Design review of the part built by this model. Coordinates are the model's own, in mm. Coordinates: 2 decimals unless noted, no trailing zeros. Loops run counter-clockwise (first coordinate to the right, second up) from the corner with the lowest first, then second, coordinate; pieces in that order, holes last.
Q1. Wall thickness on probe 1 along Z at (x, y) = (-20, 1.8); probe 2 along Z at (x, y) = (-1, 2.9); probe 3 along X at (y, z) = (2.3, -12): over which ranges is each line inside the solid? List them lowest first.
Q2. Add section A-A on z = 0. Give the boundary of the cut face in (x, y) (1 decimal), and give its area (3 significant figures).
Q3. Add section B-B on y = 2.35. Give the number of separate pieces and of enclosed holes in the cut face, and give its area (3 significant figures).
Q4. Draft analysis for pull direction Z (two halves, no side actions). For faces 1 (the face through (0.628, 1.565, -14.274)), 2 (the face through (0, 2, -19.05)), 3 (the face through (-12, 0, -9)), state which applies: released by +Z, released by -Z, zero draft, split by the parting line, or undercut.
Q5. Add section D-D on z = 7. Give the boundary of the cut face in (x, y) (3 decimals), and give its area (3 significant figures).
Q6. Add section C-C on x = 20.32. Give the boundary of the cut face in (y, z) (3 decimals).
```python
from build123d import *

# Parameters (mm, degrees)
SKETCH1_W               = 50.8
SKETCH1_H               = 38.1
SKETCH1_R               = 14.2875
BOSS_EXTRUDE1_DEPTH     = 3.175
F_1_4_CLEARANCE_HOLE1_D = 6.7564


with BuildPart() as part:
    # Sketch1 → Boss-Extrude1 (new body)
    with BuildSketch(Plane(origin=(0, 0, 0), x_dir=(1, 0, 0), z_dir=(0, 1, 0))):
        Rectangle(SKETCH1_W, SKETCH1_H)
        with Locations(Location((0, 0, 0), (0, 0, 270))):
            Circle(SKETCH1_R, mode=Mode.SUBTRACT)
    extrude(amount=BOSS_EXTRUDE1_DEPTH)

    # 1/4 Clearance Hole1 (through all)
    with Locations(Plane(origin=(0, 3.175, 0), x_dir=(1, 0, 0), z_dir=(0, 1, 0))):
        with Locations((20.32, 0), (-19.812, 0)):
            Hole(F_1_4_CLEARANCE_HOLE1_D / 2)


solid = part.part
```
Entries:
1. probe 1: z = -19.05 to -3.37, 3.37 to 19.05
1. probe 2: z = -19.05 to -14.25, 14.25 to 19.05
1. probe 3: x = -25.4 to -7.75, 7.75 to 25.4
2. outline: (-25.4, 0) - (-23.2, 0) - (-23.2, 3.2) - (-25.4, 3.2) - close; (-16.4, 0) - (-14.3, 0) - (-14.3, 3.2) - (-16.4, 3.2) - close; (14.3, 0) - (16.9, 0) - (16.9, 3.2) - (14.3, 3.2) - close; (23.7, 0) - (25.4, 0) - (25.4, 3.2) - (23.7, 3.2) - close
2. area: 27.7 mm2
3. separate pieces: 1
3. enclosed holes: 3
3. area: 1,220 mm2
4. face 1: undercut
4. face 2: released by -Z
4. face 3: zero draft
5. outline: (-25.4, 0) - (-12.455, 0) - (-12.455, 3.175) - (-25.4, 3.175) - close; (12.455, 0) - (25.4, 0) - (25.4, 3.175) - (12.455, 3.175) - close
5. area: 82.2 mm2
6. outline: (0, -19.05) - (3.175, -19.05) - (3.175, -3.378) - (0, -3.378) - close; (0, 3.378) - (3.175, 3.378) - (3.175, 19.05) - (0, 19.05) - close
